Input: part model. Units: mm. Frame: model coordinates. Face numbers are marked on the shaded views. Round coordinates to 2 decimals unless told otherwise and drop trailing zeros. Loops run counter-clockwise (first coordinate to the right, second up) from the corner with the lowest first, then second, coordinate; pieces in that order, holes last. Notation, with made-up numbers: (50, -5.5) -> (100, -5.5) arc R12 cw to (100, 1.5) -> close; hole circle Ø5 at (-21, 30). An arc over 180 degrees is marked (long way). Answer as a JSON object with one key per item and string values. Group by question number.
Item 1: Material intervals for line 1 (Z direction, x = 26, y = 20); line 2 (X direction, y = 21, z = 1.5); line 3 (X direction, y = 47, z = 3.15), sorted ascending. Write a range as [from, to].
Item 2: Section query B-B on y = 40. Return loops of the section in (x, z), and give its area (3 significant figures).
Item 3: Pin query (flat end, axial travel): pin 1 (15 mm diameter, centred on x = 40.5, y = 28.5, fed in from +Z); pin 2 (12 mm diameter, centred on x = 49, y = 7, fed in from +Z); pin 3 (1 mm diameter, centred on x = 18.5, z = 2, fed in from -Y). Return the tip coordinate at first contact, or that it passes through.
Item 4: Section query C-C on x = 6. Return loops of the section in (y, z).
Item 5: Draft query along X for the marked faces 1 and 2. Return one class per face: released by +X, released by -X, zero draft, split by the parting line, or undercut.
Item 6: Section query A-A on z = 3.1. Return loops of the section in (x, y), and give its area (3 significant figures).
Autodesk Inventor part; units mm, degrees
ref_plane "YZ Plane" through (0, 0, 0) normal (1, 0, 0) x (0, 1, 0)
ref_plane "XZ Plane" through (0, 0, 0) normal (0, 1, 0) x (-1, 0, 0)
ref_plane "XY Plane" through (0, 0, 0) normal (0, 0, 1) x (1, 0, 0)
sketch "Sketch1" plane through (0, 0, 0) normal (0, 0, 1) x (1, 0, 0)
  line L0 (0, 0) -> (55.88, 0)
  line L1 (55.88, 0) -> (55.88, 50.8)
  line L2 (55.88, 50.8) -> (0, 50.8)
  line L3 (0, 50.8) -> (0, 0)
  dimension "d0" = 55.88
  dimension "d1" = 50.8
extrude "Extrusion1" add sketch "Sketch1" along normal blind 3.81
sketch "Sketch2" plane through (0, 0, 0) normal (0, -1, 0) x (1, 0, 0)
  line L0 (0, 3.81) -> (55.88, 3.81)
  line L1 (5.08, 3.81) -> (2.54, 1.27)
  line L2 (2.54, 1.27) -> (53.34, 1.27)
  line L3 (53.34, 1.27) -> (50.8, 3.81)
  line L4 (5.08, 3.81) -> (50.8, 3.81)
  line L5 (0, 0) -> (0, 3.81)
  line L6 (0, 0) -> (55.88, 0)
  line L7 (55.88, 0) -> (55.88, 3.81)
  dimension "d4" = 45
  dimension "d5" = 45
  dimension "d6" = 45.72
  dimension "d7" = 2.54
  dimension "d8" = 1.27
  dimension "d12" = 2.54
  dimension "d13" = 2.54
extrude "Extrusion2" cut sketch "Sketch2" against normal blind 50.8 contours L0 L3 L2 L1
properties part number "nano_enclosure_modular_sidelock"
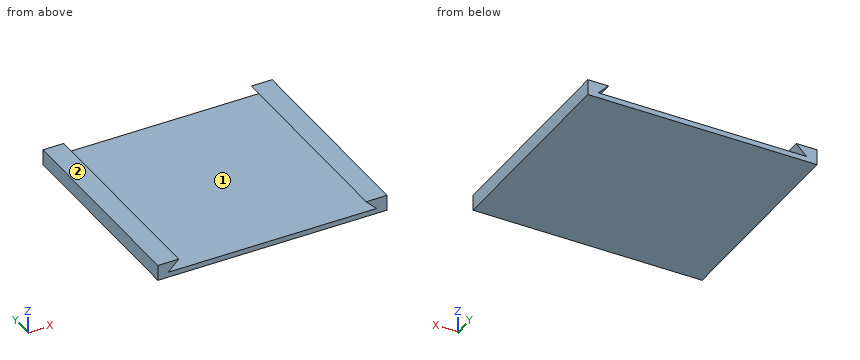
Solved:
{
 "1": {"line 1": "[0, 1.27]", "line 2": "[0, 2.77], [53.11, 55.88]", "line 3": "[0, 4.42], [51.46, 55.88]"},
 "2": {"outline": "(0, 0) -> (55.88, 0) -> (55.88, 3.81) -> (50.8, 3.81) -> (53.34, 1.27) -> (2.54, 1.27) -> (5.08, 3.81) -> (0, 3.81) -> close", "area": "90.3 mm²"},
 "3": {"pin 1": "z = 1.27", "pin 2": "z = 3.81", "pin 3": "through"},
 "4": {"outline": "(0, 0) -> (50.8, 0) -> (50.8, 1.27) -> (0, 1.27) -> close"},
 "5": {"face 1": "undercut", "face 2": "zero draft"},
 "6": {"outline": "(0, 0) -> (4.37, 0) -> (4.37, 50.8) -> (0, 50.8) -> close; (51.51, 0) -> (55.88, 0) -> (55.88, 50.8) -> (51.51, 50.8) -> close", "area": "444 mm²"}
}
